```python
from build123d import *

# Parameters (mm, degrees)
SKETCH1_W                                      = 127
SKETCH1_H                                      = 152.4
BOSS_EXTRUDE1_DEPTH                            = 12.7
SKETCH2_R                                      = 14.2875
CUT_EXTRUDE1_DEPTH                             = 13.7
SKETCH3_R                                      = 7.9375
SKETCH3_R_2                                    = 1.016
CUT_EXTRUDE2_DEPTH                             = 13.7
SKETCH4_R                                      = 36.195
CUT_EXTRUDE3_DEPTH                             = 6.35
SKETCH5_R                                      = 19.05
CUT_EXTRUDE4_DEPTH                             = 2.54
CSK_FOR_8_FLAT_HEAD_MACHINE_SCREW1_D           = 4.4958
CSK_FOR_8_FLAT_HEAD_MACHINE_SCREW1_CSINK_D     = 8.4328
CSK_FOR_8_FLAT_HEAD_MACHINE_SCREW1_CSINK_ANGLE = 82
FILLET1_R                                      = 12.7
F_1_4_20_TAPPED_HOLE1_AT_2_COUNT               = 2
F_1_4_20_TAPPED_HOLE1_AT_2_PITCH               = 38.1
SKETCH10_W                                     = 12.7
SKETCH10_H                                     = 19.05
BOSS_EXTRUDE2_DEPTH                            = 12.7
SKETCH11_R                                     = 0.79375
CUT_EXTRUDE5_DEPTH                             = 13.7


with BuildPart() as part:
    # Sketch1 → Boss-Extrude1 (new body)
    with BuildSketch(Plane.XY):
        with Locations((0, 76.2)):
            Rectangle(SKETCH1_W, SKETCH1_H)
    extrude(amount=BOSS_EXTRUDE1_DEPTH)

    # Sketch2 → Cut-Extrude1 (cut, through all)
    with BuildSketch(Plane(origin=(0, 0, 0), x_dir=(-1, 0, 0), z_dir=(0, 0, -1))):
        with BuildLine():
            Line((44.45, 50.8), (63.5, 50.8))
            Line((63.5, 50.8), (63.5, 152.4))
            Line((63.5, 152.4), (-63.5, 152.4))
            Line((-63.5, 152.4), (-63.5, 50.8))
            Line((-63.5, 50.8), (-44.45, 50.8))
            Line((-44.45, 50.8), (-23.686198751, 104.421913036))
            ThreePointArc((-23.686198751, 104.421913036), (0, 120.65), (23.686198751, 104.421913036))
            Line((23.686198751, 104.421913036), (44.45, 50.8))
        make_face()
        with Locations((0, 95.25)):
            Circle(SKETCH2_R)
    extrude(amount=-CUT_EXTRUDE1_DEPTH, mode=Mode.SUBTRACT)

    # Sketch3 → Cut-Extrude2 (cut, through all)
    with BuildSketch(Plane.XY.offset(12.7)):
        with Locations((0, 44.45)):
            Circle(SKETCH3_R)
        with Locations((-25.019, 44.45)):
            Circle(SKETCH3_R_2)
        with Locations((25.019, 44.45)):
            Circle(SKETCH3_R_2)
        with Locations((0, 69.469)):
            Circle(SKETCH3_R_2)
        with Locations((0, 19.431)):
            Circle(SKETCH3_R_2)
    extrude(amount=-CUT_EXTRUDE2_DEPTH, mode=Mode.SUBTRACT)

    # Sketch4 → Cut-Extrude3 (cut)
    with BuildSketch(Plane.XY.offset(12.7)):
        with Locations((0, 44.45)):
            Circle(SKETCH4_R)
    extrude(amount=-CUT_EXTRUDE3_DEPTH, mode=Mode.SUBTRACT)

    # Sketch5 → Cut-Extrude4 (cut)
    with BuildSketch(Plane.XY.offset(6.35)):
        with Locations((0, 44.45)):
            Circle(SKETCH5_R)
    extrude(amount=-CUT_EXTRUDE4_DEPTH, mode=Mode.SUBTRACT)

    # CSK for #8 Flat Head Machine Screw1 (through all)
    with Locations(Plane(origin=(0, 0, 0), x_dir=(-1, 0, 0), z_dir=(0, 0, -1))):
        with Locations((0, 69.469), (25.019, 44.45), (0, 19.431), (-25.019, 44.45)):
            CounterSinkHole(CSK_FOR_8_FLAT_HEAD_MACHINE_SCREW1_D / 2, CSK_FOR_8_FLAT_HEAD_MACHINE_SCREW1_CSINK_D / 2, counter_sink_angle=CSK_FOR_8_FLAT_HEAD_MACHINE_SCREW1_CSINK_ANGLE)

    # Fillet1
    fillet1_edges = [part.edges().sort_by_distance(p)[0] for p in [
        (44.45, 50.8, 6.35),
        (-44.45, 50.8, 6.35),
    ]]
    fillet(fillet1_edges, radius=FILLET1_R)

    # Sketch8 → 1/4-20 Tapped Hole1 (revolve, cut)
    with BuildSketch(Plane(origin=(63.5, 44.45, 6.35), x_dir=(0, 0, -1), z_dir=(0, 1, 0))):
        Polygon((0, 0), (0, 18.043816902), (2.5527, 16.51), (2.5527, 0), align=None)
    f_1_4_20_tapped_hole1 = revolve(axis=Axis((69.85, 44.45, 6.35), (-1, 0, 0)), mode=Mode.SUBTRACT)

    # 1/4-20 Tapped Hole1 at 2: 1/4-20 Tapped Hole1 ×2
    with Locations(*[(0, -i * F_1_4_20_TAPPED_HOLE1_AT_2_PITCH, 0) for i in range(1, F_1_4_20_TAPPED_HOLE1_AT_2_COUNT)]):
        add(f_1_4_20_tapped_hole1, mode=Mode.SUBTRACT)

    # Sketch10 → Boss-Extrude2 (add)
    with BuildSketch(Plane(origin=(63.5, 0, 0), x_dir=(0, 0, -1), z_dir=(1, 0, 0))):
        with Locations((-6.35, 25.4)):
            Rectangle(SKETCH10_W, SKETCH10_H)
    boss_extrude2 = extrude(amount=BOSS_EXTRUDE2_DEPTH)

    # Sketch11 → Cut-Extrude5 (cut, through all)
    with BuildSketch(Plane.XY.offset(12.7)):
        with Locations((63.5, 35.71875)):
            Circle(SKETCH11_R)
        with Locations((63.5, 15.08125)):
            Circle(SKETCH11_R)
    cut_extrude5 = extrude(amount=-CUT_EXTRUDE5_DEPTH, mode=Mode.SUBTRACT)

    # Mirror1: 1/4-20 Tapped Hole1, Boss-Extrude2, Cut-Extrude5 across plane
    add(f_1_4_20_tapped_hole1.mirror(Plane(origin=(0, 0, 0), x_dir=(0, 0, 1), z_dir=(1, 0, 0))), mode=Mode.SUBTRACT)
    add(boss_extrude2.mirror(Plane(origin=(0, 0, 0), x_dir=(0, 0, 1), z_dir=(1, 0, 0))))
    add(cut_extrude5.mirror(Plane(origin=(0, 0, 0), x_dir=(0, 0, 1), z_dir=(1, 0, 0))), mode=Mode.SUBTRACT)

    # Mirror1 copy 1 sketch → Mirror1 copy 1 (revolve, cut)
    with BuildSketch(Plane(origin=(-63.5, 6.35, 6.35), x_dir=(0, 0, -1), z_dir=(0, 1, 0))):
        Polygon((0, 0), (0, -18.043816902), (2.5527, -16.51), (2.5527, 0), align=None)
    revolve(axis=Axis((-69.85, 6.35, 6.35), (-1, 0, 0)), mode=Mode.SUBTRACT)


solid = part.part
```
For this review, take the finished solid that the model builds, in its own axes (mm). A direction names the side the tool comes from. Coordinates: 2 decimals unless noted, no trailing zeros. Order: outer loops, then holes, each group sorted by start corner. A loop starts at its lowest first (then second) coordinate and runs counter-clockwise, first axis right, second up. Notation, with made-up numbers: (-19, 80) -> (33, 80) arc R20 cw to (33, 109) -> close; hole circle Ø6 at (-31, 12). An arc over 180 degrees is marked (long way). Answer as CSV lines item,"result".
Q1. We need section C-C (y = 29.5). State the section outline as (x, z) points.
Model answer:
outline,"(-76.2, 0) -> (76.2, 0) -> (76.2, 12.7) -> (32.96, 12.7) -> (32.96, 6.35) -> (11.81, 6.35) -> (11.81, 3.81) -> (-11.81, 3.81) -> (-11.81, 6.35) -> (-32.96, 6.35) -> (-32.96, 12.7) -> (-76.2, 12.7) -> close"
Q2. We need section A-A (z = 11). Count the separate pieces of the cut face and the enclosed holes in it, plus the area to 3 significant figures.
Model answer:
separate pieces,"1"
enclosed holes,"2"
area,"6,410 mm2"
Q3. We need section B-B (x = 57). State the section outline as (y, z) points, plus the area to 3 significant figures.
Model answer:
outline,"(0, 0) -> (50.8, 0) -> (50.8, 12.7) -> (0, 12.7) -> close; hole circle Ø5.11 at (6.35, 6.35); hole circle Ø5.11 at (44.45, 6.35)"
area,"604 mm2"
Q4. For faces 4 (the face through (70, 15.875, 6)), 5 (the face through (55.36, 41.92, 6.68)), 6 (the face through (-55.361, 4.198, 4.978)), list the 3-axis set-ups (+Z, -Z, +X, -X, +Y, -Y) from which the entire face can be reached by the end or side of a thin tool; tool diameter is ignored.
Model answer:
face 4,"+Z, -Z, +X, -Y"
face 5,"+X"
face 6,"-X"
Q5. Wall thickness on line 1 along Y through (x, z) = (0, 5.3); line 2 along Y through (x, z) = (59, 6.35); line 3 along X through (y, z) = (19.5, 4): over which ranges is each line inside the solid? List them lowest first. Write a range as [from, to].
Model answer:
line 1,"y = [0, 17.18], [21.68, 25.4], [63.5, 67.22], [71.72, 80.96], [109.54, 120.65]"
line 2,"y = [0, 3.8], [8.9, 41.9], [47, 50.8]"
line 3,"x = [-76.2, -2.25], [2.25, 76.2]"
Q6. We need section D-D (x = 38.5). State the section outline as (y, z) points, plus the area to 3 significant figures.
Model answer:
outline,"(0, 0) -> (66.17, 0) -> (66.17, 12.7) -> (0, 12.7) -> close"
area,"840 mm2"
Q7. Draft analysis for pull direction Y (two halves, no side actions). For faces 1 (the face through (-45.72, 6.33, 6.79)), 2 (the face through (58, 50.8, 6)), 3 (the face through (-1, 0, 6)), state which applies: released by +Y, released by -Y, zero draft, split by the parting line, or undercut.
Model answer:
face 1,"undercut"
face 2,"released by +Y"
face 3,"released by -Y"
Q8. Clearance check with flat-ended pins moving along their axes: pin 1 Ø4 at (x, z) = (72.5, 4.5) entering from +Y (3 decimals); pin 2 Ø3 at (y, z) = (76.5, 9.5) entering from -X; pin 3 Ø3 at (y, z) = (98, 1.5) entering from +X. State where each tip first meets the part, or that it passes through.
Model answer:
pin 1,"stops at y = 34.925"
pin 2,"stops at x = -35.08"
pin 3,"stops at x = 26.75"
